Geometry check sheet. Reference: the model listing, model coordinates, mm. A direction names the side the tool comes from. Give positions to 0.01 mm unless a question says otherwise; leave off trailing zeros. Write each loop counter-clockwise with the first axis right and the second up, starting at its lowest first coordinate (ties: lowest second). Pieces come first, ordered by that corner, then holes. Notation, with made-up numbers: M 86.5,64 L 96.5,64 A24 ccw 96.5,87 Z; hole C -22.75,59 d8. An arc over 180 degrees is marked long. Use one line per item in the form item = value. Start each with the question number.
```python
from build123d import *

# Parameters (mm, degrees)
SKETCH_W        = 144
SKETCH_H        = 144
PAD_DEPTH       = 37
SKETCH001_W     = 130
SKETCH001_H     = 130
POCKET_DEPTH    = 37.001
SKETCH002_W     = 130
SKETCH002_H     = 34
POCKET001_DEPTH = 144.001
SKETCH003_W     = 130
SKETCH003_H     = 34
POCKET002_DEPTH = 144.001
SKETCH004_W     = 144
SKETCH004_H     = 144
POCKET003_DEPTH = 1.5


with BuildPart() as part:
    # Sketch → Pad (new body)
    with BuildSketch(Plane.XY):
        Rectangle(SKETCH_W, SKETCH_H)
    extrude(amount=PAD_DEPTH)

    # Sketch001 (on Face6 of Pad) → Pocket (cut, through all)
    with BuildSketch(Plane.XY.offset(37)):
        Rectangle(SKETCH001_W, SKETCH001_H)
    extrude(amount=-POCKET_DEPTH, mode=Mode.SUBTRACT)

    # Sketch002 (on Face3 of Pocket) → Pocket001 (cut, through all)
    with BuildSketch(Plane.YZ.offset(72)):
        with Locations((0, 17)):
            Rectangle(SKETCH002_W, SKETCH002_H)
    extrude(amount=-POCKET001_DEPTH, mode=Mode.SUBTRACT)

    # Sketch003 (on Face8 of Pocket001) → Pocket002 (cut, through all)
    with BuildSketch(Plane(origin=(0, 72, 0), x_dir=(-1, 0, 0), z_dir=(0, 1, 0))):
        with Locations((0, 17)):
            Rectangle(SKETCH003_W, SKETCH003_H)
    extrude(amount=-POCKET002_DEPTH, mode=Mode.SUBTRACT)

    # Sketch004 → Pocket003 (cut, symmetric)
    with BuildSketch(Plane.XY):
        Rectangle(SKETCH004_W, SKETCH004_H)
    extrude(amount=POCKET003_DEPTH, both=True, mode=Mode.SUBTRACT)


solid = part.part
```
(1) Draft check along Y on faces 1 (the flat face through (0, -72, 35)), 2 (the flat face through (69, -1, 34)), 3 (the flat face through (-69, 69, 1.5)). Enter one of: released by +Y, released by -Y, zero draft, split by the parting line, or undercut.
(2) Depth check by flat-ended pin: pin 1 (7.5 mm diameter, centred on x = -29, y = -69, fed in from -Z). Enter the tip coordinate at first touch or a pass-through.
(3) Sectioned sample at A-A, the plane y = 36. Record the boundary of the cut face in (x, z).
(4) Tool access check on faces 4 (the flat face through (65, -68, 18)), 5 (the flat face through (68, 69, 1.5)), 6 (the flat face through (-68, -65, 18)). Record the directions out of +Z, -Z, +X, -X, +Y, -Y that give a thin tool (end or side, any length) a straight path to the whole face; none if there is none.
(5) Sectioned sample at B-B, the plane z = 28. Record the boundary of the cut face in (x, y), plus the area to 3 significant figures.
Numbers:
q1.face_1 = released by -Y
q1.face_2 = undercut
q1.face_3 = zero draft
q2.pin_1 = 34
q3.outline = M -72,34 L -65,34 L -65,37 L -72,37 Z; M 65,34 L 72,34 L 72,37 L 65,37 Z
q4.face_4 = -Z, +Y, -Y
q4.face_5 = -Z, +X, -X, +Y, -Y
q4.face_6 = -Z, +X, -X
q5.outline = M -72,-72 L -65,-72 L -65,-65 L -72,-65 Z; M -72,65 L -65,65 L -65,72 L -72,72 Z; M 65,-72 L 72,-72 L 72,-65 L 65,-65 Z; M 65,65 L 72,65 L 72,72 L 65,72 Z
q5.area = 196 mm2
